Source: three-view drawing plus pictorial views. Frame: mm from the lowest corner of the part. A direction names the side the tool comes from. Round coordinates to 2 decimals unless told otherwise and drop trailing zeros. Write each loop counter-clockwise with the first axis right and the second up, starting at its lowest first coordinate (ties: lowest second). Pieces come first, ordered by that corner, then holes.
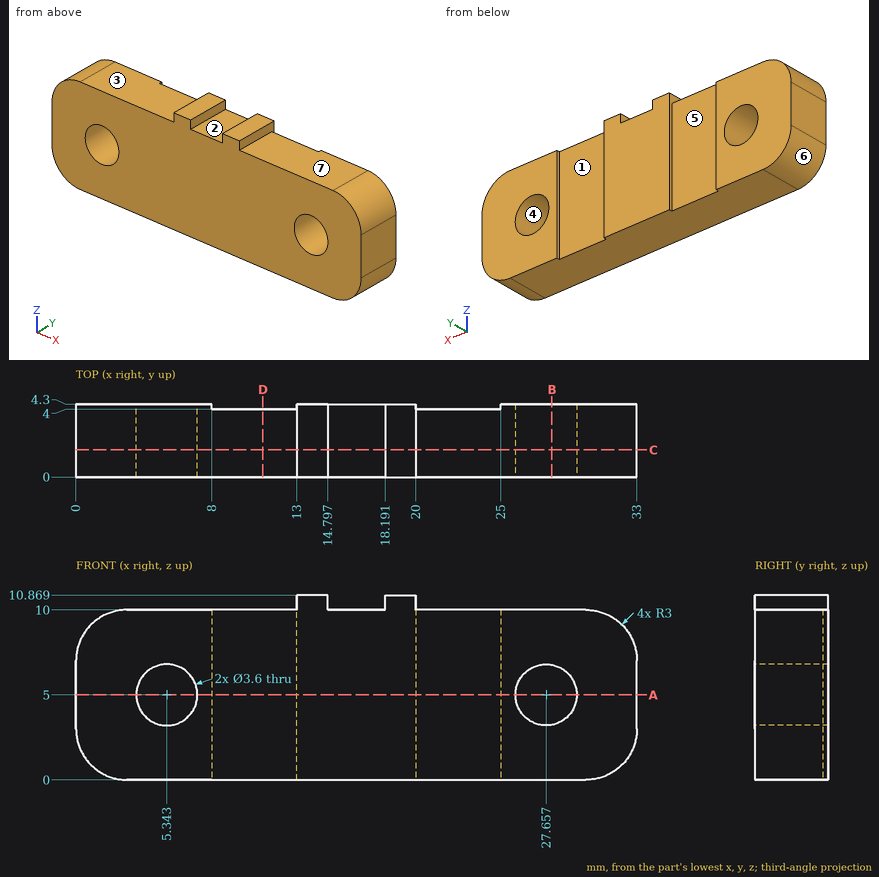
1) Section D-D on x = 11. Output: boundary loops of the cut face in (y, z), plus the area to 3 significant figures.
2) Draft query along Z for the marked faces 4, 5, 6 and 7. Return one class per face: pulls with the +Z half, pulls with the -Z half, needs draft (parallel to the pull), parting line crosses it, or undercut.
3) Section A-A on z = 5. Output: boundary loops of the cut face in (x, y), plus the area to 3 significant figures.
4) Reachability of the marked faces 1, 2 and 3 from +Z, -Z, +X, -X, +Y, -Y: full face, straight path, thin tool, end or side. Return the list, or none.
5) Section B-B on x = 28. Output: boundary loops of the cut face in (y, z), plus the area to 3 significant figures.
6) Line query: probe 1 along X at (y, z) = (3.35, 5); probe 2 along X at (y, z) = (2.65, 3.75); probe 3 along Z at (x, y) = (11.5, 2.6). Output: solid intervals per line, ascending.
7) First-contact query: P1, Ø0.7, axis at y = 2, z = 10, coming from the +X side (1 decimal); P2, Ø2, axis at x = 5.343, z = 5, coming from the +Y side; P3, Ø1.3, axis at x = 10, y = 3, coming from the +Z side; P4, Ø2, axis at y = 1, z = 9.5, coming from the +X side. Flat tips, straight axial feed; report the tip coordinate or a pass-through.
8) Section C-C on y = 1.6. Output: boundary loops of the cut face in (x, z), plus the area to 3 significant figures.
Filled in:
1. outline: (0, 0) - (4, 0) - (4, 10) - (0, 10) - close
1. area: 40.0 mm2
2. face 4: undercut
2. face 5: needs draft
2. face 6: pulls with the -Z half
2. face 7: pulls with the +Z half
3. outline: (0, 0) - (3.54, 0) - (3.54, 4.3) - (0, 4.3) - close; (7.14, 0) - (25.86, 0) - (25.86, 4.3) - (25, 4.3) - (25, 4) - (20, 4) - (20, 4.3) - (13, 4.3) - (13, 4) - (8, 4) - (8, 4.3) - (7.14, 4.3) - close; (29.46, 0) - (33, 0) - (33, 4.3) - (29.46, 4.3) - close
3. area: 108 mm2
4. face 1: +Z, -Z, +Y
4. face 2: +Z, +Y, -Y
4. face 3: +Z, -X, +Y, -Y
5. outline: (0, 0) - (4.3, 0) - (4.3, 3.23) - (0, 3.23) - close; (0, 6.77) - (4.3, 6.77) - (4.3, 10) - (0, 10) - close
5. area: 27.8 mm2
6. probe 1: x = 0 to 3.54, 7.14 to 25.86, 29.46 to 33
6. probe 2: x = 0 to 4.05, 6.64 to 26.36, 28.95 to 33
6. probe 3: z = 0 to 10
7. P1: stops at x = 31.4
7. P2: passes through
7. P3: stops at z = 10
7. P4: stops at x = 32.6
8. outline: (0, 3) arc R3 ccw to (3, 0) - (30, 0) arc R3 ccw to (33, 3) - (33, 7) arc R3 ccw to (30, 10) - (20, 10) - (20, 10.87) - (18.19, 10.87) - (18.19, 10) - (14.8, 10) - (14.8, 10.87) - (13, 10.87) - (13, 10) - (3, 10) arc R3 ccw to (0, 7) - close; hole circle Ø3.6 at (5.34, 5); hole circle Ø3.6 at (27.66, 5)
8. area: 305 mm2
